from build123d import *

# Parameters (mm, degrees)
F0_W     = 7.62
F0_H     = 7.62
F0_R     = 3.175
F1_DEPTH = 7.62
F2_R     = 3.175
F3_DEPTH = 1.27


with BuildPart() as f1:
    # F0 (on Front) → F1 (new body)
    with BuildSketch(Plane.XZ):
        Rectangle(F0_W, F0_H)
        Circle(F0_R, mode=Mode.SUBTRACT)
    extrude(amount=F1_DEPTH)

    # F2 (on face) → F3 (join)
    with BuildSketch(Plane(origin=(0, 0, -3.81), x_dir=(1, 0, 0), z_dir=(0, 0, -1))):
        with Locations((0, 3.81)):
            Circle(F2_R)
    extrude(amount=F3_DEPTH)


solid = f1.part
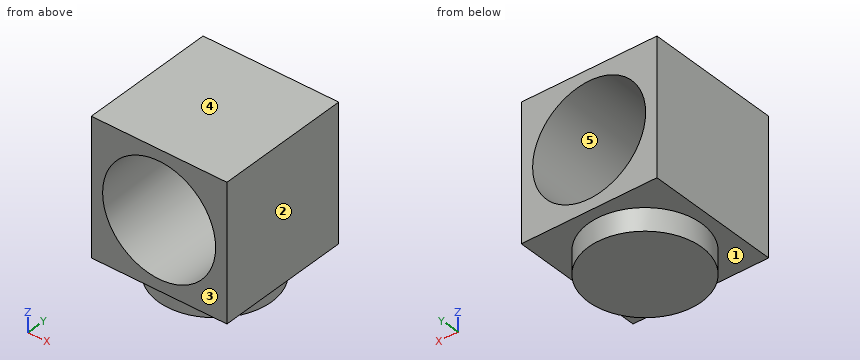
CAD build for the part. Positions are in the model's coordinates, mm. Face numbers are marked on the shaded views. A direction names the side the tool comes from. Give positions to 0.01 mm unless a question says otherwise; leave off trailing zeros. Loops run counter-clockwise (first coordinate to the right, second up) from the corner with the lowest first, then second, coordinate; pieces in that order, holes last. Notation, with made-up numbers: M 64,-21 L 99,-21 A36 ccw 99,15 Z; hole C 0.25,33.5 d8. An arc over 180 degrees is marked long. Write each question's results on one line, items separated by ' | '.
Q1. Probe probe 1 along Z at (x, y) = (0, -5.5) (3 decimals); probe 2 along X at (y, z) = (-4.75, 1.5); probe 3 along Z at (x, y) = (-2.25, -1). List the from-to ranges inside material, lowest first.
Geometry check:
probe 1: z = -5.08 to -3.175, 3.175 to 3.81 | probe 2: x = -3.81 to -2.8, 2.8 to 3.81 | probe 3: z = -3.81 to -2.24, 2.24 to 3.81
Q2. Mould opens along Z. For the marked faces 3, 4 and 5 say: pulls with the +Z half, pulls with the -Z half, needs draft (parallel to the pull), parting line crosses it, or undercut.
Geometry check:
face 3: needs draft | face 4: pulls with the +Z half | face 5: undercut
Q3. Band-saw the part on B-B on x = 0. Write the cut outline in (y, z) (3 decimals), and give its area (3 significant figures).
Geometry check:
outline: M -7.62,-3.81 L -6.985,-3.81 L -6.985,-5.08 L -0.635,-5.08 L -0.635,-3.81 L 0,-3.81 L 0,-3.175 L -7.62,-3.175 Z; M -7.62,3.175 L 0,3.175 L 0,3.81 L -7.62,3.81 Z | area: 17.7 mm²
Q4. Band-saw the part on C-C on y = -3.81. Write the cut outline in (x, z) (3 decimals).
Geometry check:
outline: M -3.81,-3.81 L -3.175,-3.81 L -3.175,-5.08 L 3.175,-5.08 L 3.175,-3.81 L 3.81,-3.81 L 3.81,3.81 L -3.81,3.81 Z; hole C 0,0 d6.35
Q5. Which spindle directions (+Z, -Z, +X, -X, +Y, -Y) get a long thin tool onto all of the face, cutting with end or side? Do the marked faces 1 and 2. Say none if no direction does.
Geometry check:
face 1: -Z | face 2: +Z, -Z, +X, +Y, -Y
Q6. Band-saw the part on A-A on z = 0. Write the cut outline in (x, y) (3 decimals), and give its area (3 significant figures).
Geometry check:
outline: M -3.81,-7.62 L -3.175,-7.62 L -3.175,0 L -3.81,0 Z; M 3.175,-7.62 L 3.81,-7.62 L 3.81,0 L 3.175,0 Z | area: 9.68 mm²
Q7. Band-saw the part on D-D on x = 3. Write the cut outline in (y, z).
Geometry check:
outline: M -7.62,-3.81 L -4.85,-3.81 L -4.85,-5.08 L -2.77,-5.08 L -2.77,-3.81 L 0,-3.81 L 0,-1.04 L -7.62,-1.04 Z; M -7.62,1.04 L 0,1.04 L 0,3.81 L -7.62,3.81 Z
